Check sheet for the modelled part. Datum: model origin and axes. Units: mm. A direction names the side the tool comes from. Give positions to 0.01 mm unless a question says otherwise; leave off trailing zeros. Order: outer loops, then holes, each group sorted by start corner. A loop starts at its lowest first (then second) coordinate and runs counter-clockwise, first axis right, second up.
from build123d import *

# Parameters (mm, degrees)
F1_DEPTH       = 20
F2_SIZE        = 20
F3_W           = 60
F3_H           = 34.6410161514
F4_DEPTH       = 20
F5_SIZE        = 2
F7_D           = 5.5
F7_CBORE_D     = 9.75
F7_CBORE_DEPTH = 5
F9_D           = 8.8
F9_DEPTH       = 51.35
F9_TIP         = 2.6437867237


with BuildPart() as f1:
    # F0 (on Top) → F1 (new body)
    with BuildSketch(Plane.XY):
        Polygon((0, 115.4700538379), (-100, -57.735026919), (100, -57.735026919), align=None)
        Polygon((-48.0384757729, -27.735026919), (0, 55.4700538379), (48.0384757729, -27.735026919), align=None, mode=Mode.SUBTRACT)
    extrude(amount=F1_DEPTH)

    # F2
    f2_edges = [f1.edges().sort_by_distance(p)[0] for p in [
        (-100, -57.735027, 10),
        (100, -57.735027, 10),
        (0, 115.470054, 10),
    ]]
    chamfer(f2_edges, length=F2_SIZE)

    # F3 (on face) → F4 (join, through all)
    with BuildSketch(Plane(origin=(0, 0, 0), x_dir=(1, 0, 0), z_dir=(0, 0, -1))):
        with Locations((0, -80.8290376865)):
            Rectangle(F3_W, F3_H)
        Polygon((70, 5.7735026919), (100, 23.0940107676), (70, 75.0555349947), (40, 57.735026919), align=None)
        Polygon((-40, 57.735026919), (-70, 75.0555349947), (-100, 23.0940107676), (-70, 5.7735026919), align=None)
    extrude(amount=-F4_DEPTH)

    # F5
    f5_edges = [f1.edges().sort_by_distance(p)[0] for p in [
        (85, -49.074773, 20),
        (85, -14.433757, 20),
        (50, 28.867513, 20),
        (30, 80.829038, 20),
        (0, 98.149546, 20),
        (-30, 80.829038, 20),
        (-50, 28.867513, 20),
        (-85, -14.433757, 20),
        (-85, -49.074773, 20),
        (-55, -66.395281, 20),
        (0, -57.735027, 20),
        (55, -66.395281, 20),
        (-24.019238, 13.867513, 20),
        (24.019238, 13.867513, 20),
        (0, -27.735027, 20),
        (85, -49.074773, 0),
        (85, -14.433757, 0),
        (50, 28.867513, 0),
        (30, 80.829038, 0),
        (0, 98.149546, 0),
        (-30, 80.829038, 0),
        (-50, 28.867513, 0),
        (-85, -14.433757, 0),
        (-85, -49.074773, 0),
        (-55, -66.395281, 0),
        (0, -57.735027, 0),
        (55, -66.395281, 0),
        (-24.019238, 13.867513, 0),
        (24.019238, 13.867513, 0),
        (0, -27.735027, 0),
        (100, -23.094011, 10),
        (70, -75.055535, 10),
        (30, 98.149546, 10),
        (-30, 98.149546, 10),
        (-100, -23.094011, 10),
        (-70, -75.055535, 10),
    ]]
    chamfer(f5_edges, length=F5_SIZE)

    # F7 (through all)
    with Locations(Plane.XY.offset(20)):
        with Locations((-66.1121593217, -55.4903810568), (-81.1121593217, -29.5096189432), (-15, 85), (15, 85), (81.1121593217, -29.5096189432), (66.1121593217, -55.4903810568)):
            CounterBoreHole(F7_D / 2, F7_CBORE_D / 2, F7_CBORE_DEPTH)

    # F9
    with Locations(Plane.XZ.offset(57.735026919)):
        with Locations((0, 10)):
            Hole(F9_D / 2, depth=F9_DEPTH)
            with Locations((0, 0, -(F9_DEPTH + F9_TIP / 2))):  # 118° drill point
                Cone(0, F9_D / 2, F9_TIP, mode=Mode.SUBTRACT)


solid = f1.part
1) Draft check along Y on faces 5 (the face through (-84.332, -14.048, 9.888)), 6 (the face through (-84.804, -49.414, 9.888)), 7 (the face through (-64, -58, 15)). Enter one of: +Y half, -Y half, draft (parallel to the pull), parting line (faces both ways), or undercut.
Recorded:
face 5: +Y half
face 6: -Y half
face 7: undercut
2) Set-up check for faces 1 (the face through (-54.21, -64.77, 0.99)), 2 (the face through (-53.936, -65.781, 9.888)), 3 (the face through (-67.17, -60.25, 17.54)), 4 (the face through (-25.258, 13.75, 0.986)): record each of +Z, -Z, +X, -X, +Y, -Y from which the full face is reachable in a straight line by a thin tool's end or side.
Recorded:
face 1: -Z, -Y
face 2: +Z, -Z, -Y
face 3: +Z
face 4: -Z
3) Section check C-C, the plane z = 10. State how many separate pieces and enclosed holes the cut face has, then the cut area to 3 significant figures.
Recorded:
separate pieces: 1
enclosed holes: 6
area: 14,500 mm2
4) Section check A-A, the plane y = 85. Record the cut outline in (x, z) (3 decimals), then the cut area to 4 significant figures.
Recorded:
outline: (-30, 2) - (-28, 0) - (-17.75, 0) - (-17.75, 15) - (-19.875, 15) - (-19.875, 20) - (-28, 20) - (-30, 18) - close; (-12.25, 0) - (12.25, 0) - (12.25, 15) - (10.125, 15) - (10.125, 20) - (-10.125, 20) - (-10.125, 15) - (-12.25, 15) - close; (17.75, 0) - (28, 0) - (30, 2) - (30, 18) - (28, 20) - (19.875, 20) - (19.875, 15) - (17.75, 15) - close
area: 929.5 mm2
5) Section check B-B, the plane x = 15. Record the cut outline in (y, z) (3 decimals), then the cut area to 3 significant figures.
Recorded:
outline: (-57.735, 2) - (-55.735, 0) - (-29.735, 0) - (-27.735, 2) - (-27.735, 18) - (-29.735, 20) - (-55.735, 20) - (-57.735, 18) - close; (29.489, 2) - (33.489, 0) - (82.25, 0) - (82.25, 15) - (80.125, 15) - (80.125, 20) - (33.489, 20) - (29.489, 18) - close; (87.75, 0) - (96.15, 0) - (98.15, 2) - (98.15, 18) - (96.15, 20) - (89.875, 20) - (89.875, 15) - (87.75, 15) - close
area: 1,820 mm2
6) Depth check by flat-ended pin: pin 1 Ø12 at (y, z) = (65.5, 9) entering from +X; pin 2 Ø9 at (x, y) = (81.11, -29.51) entering from +Z; pin 3 Ø3.5 at (x, y) = (15, 85) entering from +Z; pin 4 Ø6 at (x, y) = (-50.5, 32.5) entering from -Z. Enter the tip coordinate at first touch or a pass-through.
Recorded:
pin 1: stops at x = 32.31
pin 2: stops at z = 15
pin 3: passes through
pin 4: stops at z = 1.25
7) Section check D-D, the plane y = -43.5. Record the cut outline in (x, z), then the cut area to 3 significant figures.
Recorded:
outline: (-88.22, 2) - (-85.91, 0) - (85.91, 0) - (88.22, 2) - (88.22, 18) - (85.91, 20) - (-85.91, 20) - (-88.22, 18) - close; hole circle Ø8.8 at (0, 10)
area: 3,460 mm2
8) Material ranges on L1, parallel to Y at x = 15, z = 9.5; L2, parallel to Y at x = 15, z = 16.95 (3 decimals); L3, parallel to X at y = 78.5, z = 12.75, recorded low to high.
Recorded:
L1: y = -57.74 to -27.74, 29.49 to 82.25, 87.75 to 98.15
L2: y = -57.735 to -27.735, 29.489 to 80.125, 89.875 to 98.15
L3: x = -30 to 30
